Autodesk Inventor part; units mm, degrees
ref_plane "Work Plane1" through (6, 0, 0) normal (0, 0.5, 0.866) x (1, 0, 0)
ref_plane "YZ Plane" through (0, 0, 0) normal (1, 0, 0) x (0, 1, 0)
ref_plane "XZ Plane" through (0, 0, 0) normal (0, 1, 0) x (-1, 0, 0)
sketch "Sketch1" plane through (0, 0, 0) normal (0, 0, 1) x (1, 0, 0)
  line L0 (1.0774, 0) -> (12, 0)
  line L1 (12, 0) -> (12, 2)
  line L2 (12, 2) -> (0, 2)
  line L3 (0, 2) -> (0, 3.5)
  line L4 (0, 3.5) -> (-2.8, 3.5)
  line L5 (-2.8, 3.5) -> (-2.8, 1.7321)
  line L6 (-2.8, 1.7321) -> (-1.2, 1.7321)
  line L7 (-1.2, 1.7321) -> (-0.7774, 1)
  line L8 (-5.76, 0) -> (14.96, 0)
  line L9 (0, -0.7) -> (0, 4.2)
  line L10 (-0.7774, 1) -> (0.5, 1)
  line L11 (0.5, 1) -> (1.0774, 0)
  line L12 (-2.8, 1.7321) -> (-2.8, 0) construction
  line L13 (-2.8, 3.1) -> (-2.4, 3.5)
  dimension "d0" = 2.8
  dimension "d1" = 1.6
  dimension "d2" = 60
  dimension "d3" = 4
  dimension "d4" = 3.4641
  dimension "d5" = 7
  dimension "d15" = 3.3
  dimension "d16" = 2
  dimension "d17" = 12
  dimension "d32" = 45
  dimension "d33" = 0.4
revolve "Body" add sketch "Sketch1" angle 360 about axis through (1.0774, 0, 0) along (1, 0, 0) contours L11 L10 L9 L2 L1 L0 | L10 L7 L6 L5 L13 L4 L3 L9 | L13 L5 L4
revolve "Chamfer2" cut sketch "Sketch1" angle 360 about axis through (-10, 0, 0) along (1, 0, 0) contours L13 L5 L4
sketch "Sketch2" plane through (-2.8, 0, 0) normal (-1, 0, 0) x (0, 0, 1)
  circle A0 centre (0, 0) radius 1.7321
  line L0 (0, -4.9) -> (0, 4.9)
  line L1 (-4.9, 0) -> (4.9, 0)
  line L2 (1.7321, 0) -> (0.866, -1.5)
  line L3 (0.866, -1.5) -> (-0.866, -1.5)
  line L4 (-0.866, -1.5) -> (-1.7321, 0)
  line L5 (-1.7321, 0) -> (-0.866, 1.5)
  line L6 (-0.866, 1.5) -> (0.866, 1.5)
  line L7 (0.866, 1.5) -> (1.7321, 0)
extrude "Slot" add sketch "Sketch2" against normal up to next contours L7 A0 | A0 L2 | L6 L0 A0 | A0 L0 L3 | L0 L6 A0 | A0 L3 L0 | L4 A0 | A0 L5
thread "Thread"
chamfer "Chamfer1" distance 0.4294 distance2 0.4294 1 edges at (12, -2, 0) measured on face at (12, -1.1003, -0.6618)
ref_plane "Work Plane1" through (6, 0, 0) normal (0, 0.5, 0.866) x (1, 0, 0)
equation "\"d0\" = KOH"
equation "\"d1\" = INTI"
equation "\"d3\" = GD"
equation "\"d4\" = 1.1547 * SW"
equation "\"d5\" = KOD"
equation "\"d15\" = INFT"
equation "\"d16\" = SDT"
equation "\"d17\" = NLG"
equation "\"d33\" = Cham"
equation "\"d7\" = GEL"
equation "\"d9\" = -0.5 * SPD + 0.5 * GD"
equation "\"d12\" = GUL"
equation "\"GD\" = NND"
equation "\"NLG\" = 12"
equation "\"GEL\" = 8.5"
equation "\"KOD\" = 7"
equation "\"KOH\" = 2.8"
equation "\"GUL\" = 0.61345 * PTC"
equation "\"SW\" = 3"
equation "\"INTI\" = 1.6"
equation "\"SPD\" = NND - 1.2269 * PTC"
equation "\"SDT\" = 2"
equation "\"INFT\" = 3.3"
equation "\"Cham\" = 0.4"
equation "\"TOA\" = 30deg"
equation "\"GD1\" = THREADDIA - 1.2269 * PTC"
equation "\"THREADDIA\" = 4"
equation "\"BDM\" = NND"
equation "\"FAWI\" = 45deg"
equation "\"RR\" = 0.1 * NND"
equation "\"PTC\" = 0.7"
equation "\"NND\" = 4"
equation "\"FAWI1\" = 45deg"
equation "\"GAL\" = 0.61345 * PTC"
equation "\"E0\" = 1.155 * SW"
properties part number "DIN 6912 - M4 x 12" material "Steel, Mild"
Input: part model. Units: mm. Frame: model coordinates. A direction names the side the tool comes from. Give positions to 0.01 mm unless a question says otherwise; leave off trailing zeros. Loops run counter-clockwise (first coordinate to the right, second up) from the corner with the lowest first, then second, coordinate; pieces in that order, holes last. Notation, with made-up numbers: (-38.5, -24) -> (-31.5, -24) arc R19 ccw to (-31.5, 3) -> close; hole circle Ø2 at (69.5, 73). An arc over 180 degrees is marked (long way). Answer as a JSON object with one key per item and string values. Group by question number.
Item 1: Cut plane A-A, the plane x = 3.75. Return the cut outline in (y, z), and give its area (3 significant figures).
Item 2: Pin query (flat end, axial travel): P1, Ø2, axis at x = 6.5, y = -2, coming from the -Z side; P2, Ø0.5, axis at x = -1.5, z = 0.5, coming from the +Y side; P3, Ø1.5, axis at x = 1, z = -1, coming from the -Y side. Return the tip coordinate at first contact, or that it passes through.
Item 3: Reachability of faces 1 (the flat face through (-2.8, -1.3, 1.3)), 2 (the flat face through (-1.945, -0.761, -1.293)), 3 (the flat face through (0, 2, -2)) from +Z, -Z, +X, -X, +Y, -Y: full face, straight path, thin tool, end or side. Return the list, or none.
Item 4: Pull-direction query (Y, two-part tool) for faces 4 (the flat face through (12, 0, 0)), 5 (the flat face through (-1.945, 0.74, -1.305)), 6 (the conical face through (0.977, -0.138, 0.106)), 7 (the cylindrical face through (-1.217, 3.233, 1.341)); classes: released by +Y, released by -Y, zero draft, split by the parting line, or undercut.
Item 5: Line query: probe 1 along Z at (x, y) = (0.25, 0); probe 2 along Z at (x, y) = (-0.35, 0); probe 3 along X at (y, z) = (2.25, 0.5). Output: solid intervals per line, ascending.
Checks:
{
 "1": {"outline": "circle Ø4 at (0, 0)", "area": "12.6 mm²"},
 "2": {"P1": "stops at z = -1.73", "P2": "stops at y = 3.49", "P3": "stops at y = -1.98"},
 "3": {"face 1": "+Z, -Z, -X, +Y, -Y", "face 2": "-X", "face 3": "+X"},
 "4": {"face 4": "zero draft", "face 5": "undercut", "face 6": "undercut", "face 7": "split by the parting line"},
 "5": {"probe 1": "z = -2 to -1, 1 to 2", "probe 2": "z = -3.5 to -1, 1 to 3.5", "probe 3": "x = -2.8 to 0"}
}
